Geometry check sheet. Reference: drawing and pictorial views, mm from the part's lowest x, y, z. A direction names the side the tool comes from. Coordinates: 2 decimals unless noted, no trailing zeros. Loops run counter-clockwise (first coordinate to the right, second up) from the corner with the lowest first, then second, coordinate; pieces in that order, holes last. Notation, with made-up numbers: (75.5, 3) - (87.5, 3) arc R29 ccw to (87.5, 31) - close; hole circle Ø9 at (85, 13.5). An arc over 180 degrees is marked (long way). Use a Markdown table: item, result. Add a question column.
1) Sectioned sample at C-C, the plane z = 8. Enter the section's corners in (x, y).
2) Sectioned sample at D-D, the plane y = 21.15. Enter the section's corners in (x, z).
3) Go/stop test with flat-tipped pins: P1, Ø4, axis at x = 36.65, y = 36.65, coming from the +Z side; P2, Ø10, axis at x = 37, y = 34, coming from the -Z side; P3, Ø3.5, axis at x = 12.1, z = 8, coming from the -Y side. Record where each tip stops, or that it passes through.
4) Thickness scan on line 1 (Z direction, x = 12.1, y = 46.5); line 2 (Y direction, x = 5, z = 36); line 3 (Z direction, x = 36.5, y = 35). Record the ranges inside material, lowest first.
5) Tool access check on the marked faces 1 and 2. Record the directions out of +Z, -Z, +X, -X, +Y, -Y that give a thin tool (end or side, any length) a straight path to the whole face; none if there is none.
6) Sectioned sample at A-A, the plane y = 36.65. Enter the section's corners in (x, z), then the cut area to 3 significant figures.
7) Sectioned sample at B-B, the plane x = 21.15. Enter the section's corners in (y, z), then the cut area to 3 significant figures.
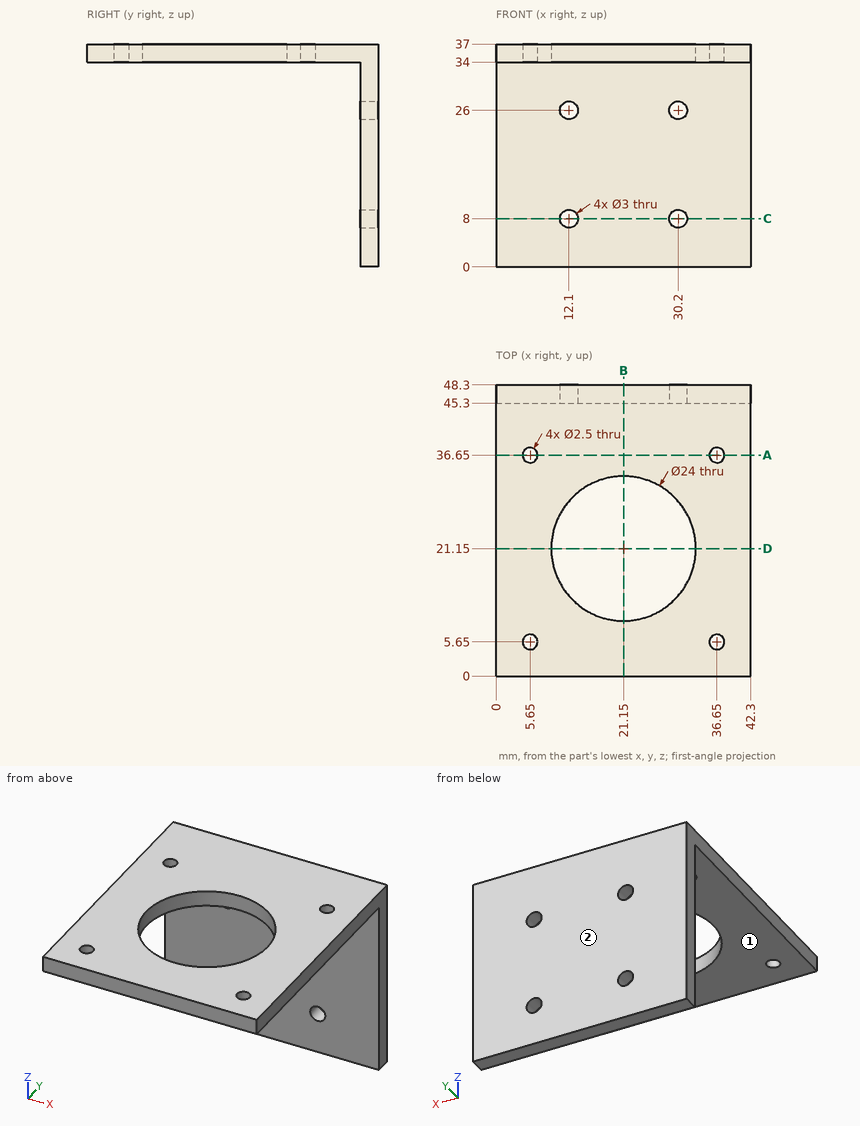
Solved:
| question | item | result |
|---|---|---|
| 1 | outline | (0, 45.3) - (10.6, 45.3) - (10.6, 48.3) - (0, 48.3) - close; (13.6, 45.3) - (28.7, 45.3) - (28.7, 48.3) - (13.6, 48.3) - close; (31.7, 45.3) - (42.3, 45.3) - (42.3, 48.3) - (31.7, 48.3) - close |
| 2 | outline | (0, 34) - (9.15, 34) - (9.15, 37) - (0, 37) - close; (33.15, 34) - (42.3, 34) - (42.3, 37) - (33.15, 37) - close |
| 3 | P1 | stops at z = 37 |
| 3 | P2 | stops at z = 34 |
| 3 | P3 | stops at y = 45.3 |
| 4 | line 1 | z = 0 to 6.5, 9.5 to 24.5, 27.5 to 37 |
| 4 | line 2 | y = 0 to 4.58, 6.72 to 35.58, 37.72 to 48.3 |
| 4 | line 3 | z = 34 to 37 |
| 5 | face 1 | -Z, +X, -X, -Y |
| 5 | face 2 | +Z, -Z, +X, -X, +Y |
| 6 | outline | (0, 34) - (4.4, 34) - (4.4, 37) - (0, 37) - close; (6.9, 34) - (35.4, 34) - (35.4, 37) - (6.9, 37) - close; (37.9, 34) - (42.3, 34) - (42.3, 37) - (37.9, 37) - close |
| 6 | area | 112 mm2 |
| 7 | outline | (0, 34) - (9.15, 34) - (9.15, 37) - (0, 37) - close; (33.15, 34) - (45.3, 34) - (45.3, 0) - (48.3, 0) - (48.3, 37) - (33.15, 37) - close |
| 7 | area | 175 mm2 |
